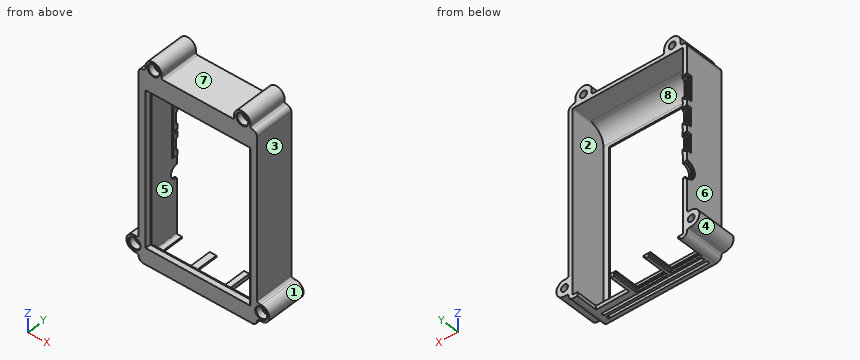
from build123d import *

# Parameters (mm, degrees)
BASE_DEPTH                      = 20.75
SHELL_T                         = -2
CLAMPS_DEPTH                    = 20.75
CLAMP_FILLETS_R                 = 1
SKETCH20_R                      = 1.8
CLAMP_HOLES_DEPTH               = 123.621878146
SKETCH21_R                      = 2.9
CLAMP_COUNTERSINKS_DEPTH        = 3.4
CLAMP_COUNTERSINK_CHAMFERS_SIZE = 0.3
SKETCH24_W                      = 14.5
SKETCH24_H                      = 12.8
USB_CUTOUT_DEPTH                = 18.25
SKETCH25_W                      = 16.5
SKETCH25_H                      = 13.5
USB_APPROACH_DEPTH              = 1.2
SKETCH28_W                      = 17.4
SKETCH28_H                      = 11.3
RJ45_CUTOUT_DEPTH               = 22.7
SKETCH29_W                      = 15
SKETCH29_H                      = 3.2
USB_C_SUPPORT_DEPTH             = 0.5
USB_C_SUPPORT_CHAMFER_SIZE      = 0.5
SKETCH30_W                      = 13
SKETCH30_H                      = 2.7
USB_C_APPROACH_DEPTH            = 1.5
USB_C_APPROACH_CHAMFER_SIZE     = 0.5
SKETCH36_W                      = 9.8
SKETCH36_H                      = 2.48
HDMI_APPROACH_DEPTH             = 1.5
HDMI_APPROACH_CHAMFER_SIZE      = 0.5
SKETCH37_W                      = 12.8
SKETCH37_H                      = 2.98
HDMI_SUPPORT_DEPTH              = 0.5
HDMI_SUPPORT_CHAMFER_SIZE       = 0.5
HDMI_CUTOUT_DEPTH               = 1
SKETCH32_R                      = 3.5
AUDIO_CUTOUT_DEPTH              = 2
SKETCH33_R                      = 4.75
AUDIO_APPROACH_DEPTH            = 1
AUDIO_APPROACH_CHAMFER_SIZE     = 0.5
AIR_SCOOP_REACH                 = 123.517
SKETCH41_W                      = 53
SKETCH41_H                      = 1.5
VENT_DEPTH                      = 2
VENT_FILLET_R                   = 0.5
SKETCH40_W                      = 52
SKETCH40_H                      = 78
SCREEN_CUTOUT_DEPTH             = 123.621878163
CHAMFER1_SIZE                   = 1.5


with BuildPart() as part:
    # Sketch2 → Base (new body)
    with BuildSketch(Plane(origin=(0, 0, 0), x_dir=(1, 0, 0), z_dir=(0, 1, 0))):
        with BuildLine():
            Line((2.5, 0), (59.5, 0))
            ThreePointArc((59.5, 0), (61.267766953, 0.732233047), (62, 2.5))
            Line((62, 2.5), (62, 97.1))
            ThreePointArc((62, 97.1), (61.267766953, 98.867766953), (59.5, 99.6))
            Line((59.5, 99.6), (2.5, 99.6))
            ThreePointArc((2.5, 99.6), (0.732233047, 98.867766953), (0, 97.1))
            Line((0, 97.1), (0, 2.5))
            ThreePointArc((0, 2.5), (0.732233047, 0.732233047), (2.5, 0))
        make_face()
    extrude(amount=BASE_DEPTH)

    # Shell
    shell_openings = [part.faces().sort_by_distance(p)[0] for p in [
        (31, 20.75, -49.8),
    ]]
    offset(amount=SHELL_T, openings=shell_openings, kind=Kind.INTERSECTION)

    # Sketch14 → Clamps (add)
    with BuildSketch(Plane.XZ):
        with BuildLine():
            Line((-2.2, -87.6), (0, -87.6))
            Line((0, -87.6), (0, -96.1))
            Line((0, -96.1), (-2.2, -96.1))
            ThreePointArc((-2.2, -96.1), (-6.45, -91.85), (-2.2, -87.6))
        make_face()
        with BuildLine():
            Line((3.5, 2.2), (3.5, 0))
            Line((3.5, 0), (12, 0))
            Line((12, 0), (12, 2.2))
            ThreePointArc((12, 2.2), (7.75, 6.45), (3.5, 2.2))
        make_face()
        with BuildLine():
            Line((64.2, -87.6), (62, -87.6))
            Line((62, -87.6), (62, -96.1))
            Line((62, -96.1), (64.2, -96.1))
            ThreePointArc((64.2, -96.1), (68.45, -91.85), (64.2, -87.6))
        make_face()
        with BuildLine():
            Line((50, 0), (50, 2.2))
            ThreePointArc((50, 2.2), (54.25, 6.45), (58.5, 2.2))
            Line((58.5, 2.2), (58.5, 0))
            Line((58.5, 0), (50, 0))
        make_face()
    extrude(amount=-CLAMPS_DEPTH)

    # Clamp Fillets
    clamp_fillets_edges = [part.edges().sort_by_distance(p)[0] for p in [
        (0, 10.375, -96.1),
        (0, 10.375, -87.6),
        (3.5, 10.375, 0),
        (12, 10.375, 0),
        (62, 10.375, -87.6),
        (62, 10.375, -96.1),
        (50, 10.375, 0),
        (58.5, 10.375, 0),
    ]]
    fillet(clamp_fillets_edges, radius=CLAMP_FILLETS_R - 0.0001)  # a hair under: the kernel refuses the full size

    # Sketch20 → Clamp Holes (cut, through all)
    with BuildSketch(Plane.XZ):
        with Locations(Location((7.75, 2.2, 0), (0, 0, 270))):
            Circle(SKETCH20_R)
        with Locations(Location((54.25, 2.2, 0), (0, 0, 270))):
            Circle(SKETCH20_R)
        with Locations(Location((64.2, -91.85, 0), (0, 0, 270))):
            Circle(SKETCH20_R)
        with Locations(Location((-2.2, -91.85, 0), (0, 0, 270))):
            Circle(SKETCH20_R)
    extrude(amount=-CLAMP_HOLES_DEPTH, mode=Mode.SUBTRACT)

    # Sketch21 → Clamp Countersinks (cut)
    with BuildSketch(Plane.XZ):
        with Locations(Location((7.75, 2.2, 0), (0, 0, 270))):
            Circle(SKETCH21_R)
        with Locations(Location((54.25, 2.2, 0), (0, 0, 270))):
            Circle(SKETCH21_R)
        with Locations(Location((64.2, -91.85, 0), (0, 0, 270))):
            Circle(SKETCH21_R)
        with Locations(Location((-2.2, -91.85, 0), (0, 0, 270))):
            Circle(SKETCH21_R)
    extrude(amount=-CLAMP_COUNTERSINKS_DEPTH, mode=Mode.SUBTRACT)

    # Clamp Countersink Chamfers
    clamp_countersink_chamfers_edges = [part.edges().sort_by_distance(p)[0] for p in [
        (-2.2, 0, -88.95),
        (64.2, 0, -88.95),
        (54.25, 0, 5.1),
        (7.75, 0, 5.1),
    ]]
    chamfer(clamp_countersink_chamfers_edges, length=CLAMP_COUNTERSINK_CHAMFERS_SIZE)

    # Sketch24 → USB Cutout (cut)
    with BuildSketch(Plane(origin=(0, 0, -99.6), x_dir=(-1, 0, 0), z_dir=(0, 0, -1))):
        with Locations((-30, 14.35)):
            Rectangle(SKETCH24_W, SKETCH24_H)
        with Locations((-12, 14.35)):
            Rectangle(SKETCH24_W, SKETCH24_H)
    extrude(amount=-USB_CUTOUT_DEPTH, mode=Mode.SUBTRACT)

    # Sketch25 → USB Approach (cut)
    with BuildSketch(Plane(origin=(0, 0, -99.6), x_dir=(-1, 0, 0), z_dir=(0, 0, -1))):
        with Locations((-30, 14)):
            Rectangle(SKETCH25_W, SKETCH25_H)
        with Locations((-12, 14)):
            Rectangle(SKETCH25_W, SKETCH25_H)
    extrude(amount=-USB_APPROACH_DEPTH, mode=Mode.SUBTRACT)

    # Sketch28 → RJ45 Cutout (cut)
    with BuildSketch(Plane(origin=(0, 0, -99.6), x_dir=(-1, 0, 0), z_dir=(0, 0, -1))):
        with Locations((-48.75, 15.1)):
            Rectangle(SKETCH28_W, SKETCH28_H)
    extrude(amount=-RJ45_CUTOUT_DEPTH, mode=Mode.SUBTRACT)

    # Sketch29 → USB-C Support (add)
    with BuildSketch(Plane(origin=(2, 0, 0), x_dir=(0, 0, -1), z_dir=(1, 0, 0))):
        with Locations((22.55, 19.15)):
            Rectangle(SKETCH29_W, SKETCH29_H)
    extrude(amount=USB_C_SUPPORT_DEPTH)

    # USB-C Support Chamfer
    usb_c_support_chamfer_edges = [part.edges().sort_by_distance(p)[0] for p in [
        (2.5, 19.15, -30.05),
        (2.5, 17.55, -22.55),
        (2.5, 19.15, -15.05),
    ]]
    chamfer(usb_c_support_chamfer_edges, length=USB_C_SUPPORT_CHAMFER_SIZE - 0.0001)  # a hair under: the kernel refuses the full size

    # Sketch30 → USB-C Approach (cut)
    with BuildSketch(Plane.ZY):
        with Locations((-22.55, 19.4)):
            Rectangle(SKETCH30_W, SKETCH30_H)
    extrude(amount=-USB_C_APPROACH_DEPTH, mode=Mode.SUBTRACT)

    # USB-C Approach Chamfer
    usb_c_approach_chamfer_edges = [part.edges().sort_by_distance(p)[0] for p in [
        (1.5, 19.4, -29.05),
        (1.5, 19.4, -16.05),
        (1.5, 18.05, -22.55),
    ]]
    chamfer(usb_c_approach_chamfer_edges, length=USB_C_APPROACH_CHAMFER_SIZE)

    # Sketch36 → HDMI Approach (cut)
    with BuildSketch(Plane.ZY):
        with Locations((-50.85, 19.51)):
            Rectangle(SKETCH36_W, SKETCH36_H)
        with Locations((-37.35, 19.51)):
            Rectangle(SKETCH36_W, SKETCH36_H)
    extrude(amount=-HDMI_APPROACH_DEPTH, mode=Mode.SUBTRACT)

    # HDMI Approach Chamfer
    hdmi_approach_chamfer_edges = [part.edges().sort_by_distance(p)[0] for p in [
        (1.5, 19.51, -55.75),
        (1.5, 19.51, -45.95),
        (1.5, 18.27, -50.85),
        (1.5, 19.51, -42.25),
        (1.5, 19.51, -32.45),
        (1.5, 18.27, -37.35),
    ]]
    chamfer(hdmi_approach_chamfer_edges, length=HDMI_APPROACH_CHAMFER_SIZE)

    # Sketch37 → HDMI Support (add)
    with BuildSketch(Plane(origin=(2, 0, 0), x_dir=(0, 0, -1), z_dir=(1, 0, 0))):
        with Locations((37.35, 19.26)):
            Rectangle(SKETCH37_W, SKETCH37_H)
        with Locations((50.85, 19.26)):
            Rectangle(SKETCH37_W, SKETCH37_H)
    extrude(amount=HDMI_SUPPORT_DEPTH)

    # HDMI Support Chamfer
    hdmi_support_chamfer_edges = [part.edges().sort_by_distance(p)[0] for p in [
        (2.5, 19.26, -57.25),
        (2.5, 17.77, -50.85),
        (2.5, 19.26, -44.45),
        (2.5, 19.26, -43.75),
        (2.5, 17.77, -37.35),
        (2.5, 19.26, -30.95),
    ]]
    chamfer(hdmi_support_chamfer_edges, length=HDMI_SUPPORT_CHAMFER_SIZE - 0.0001)  # a hair under: the kernel refuses the full size

    # Sketch38 → HDMI Cutout (cut)
    with BuildSketch(Plane.ZY.offset(-1.5)):
        with BuildLine():
            Line((-54.25, 20.75), (-47.45, 20.75))
            Line((-47.45, 20.75), (-47.45, 20.67))
            ThreePointArc((-47.45, 20.67), (-47.713603897, 20.033603897), (-48.35, 19.77))
            Line((-48.35, 19.77), (-53.35, 19.77))
            ThreePointArc((-53.35, 19.77), (-53.986396103, 20.033603897), (-54.25, 20.67))
            Line((-54.25, 20.67), (-54.25, 20.75))
        make_face()
        with BuildLine():
            Line((-40.75, 20.75), (-33.95, 20.75))
            Line((-33.95, 20.75), (-33.95, 20.67))
            ThreePointArc((-33.95, 20.67), (-34.213603897, 20.033603897), (-34.85, 19.77))
            Line((-34.85, 19.77), (-39.85, 19.77))
            ThreePointArc((-39.85, 19.77), (-40.486396103, 20.033603897), (-40.75, 20.67))
            Line((-40.75, 20.67), (-40.75, 20.75))
        make_face()
        with BuildLine():
            Line((-27.55, 20.75), (-17.55, 20.75))
            Line((-17.55, 20.75), (-17.55, 20.713167547))
            ThreePointArc((-17.55, 20.713167547), (-17.890683887, 19.890683887), (-18.713167547, 19.55))
            Line((-18.713167547, 19.55), (-26.386832453, 19.55))
            ThreePointArc((-26.386832453, 19.55), (-27.209316113, 19.890683887), (-27.55, 20.713167547))
            Line((-27.55, 20.713167547), (-27.55, 20.75))
        make_face()
    extrude(amount=-HDMI_CUTOUT_DEPTH, mode=Mode.SUBTRACT)

    # Sketch32 → Audio Cutout (cut)
    with BuildSketch(Plane.ZY):
        with Locations((-65.35, 20.75)):
            Circle(SKETCH32_R)
    extrude(amount=-AUDIO_CUTOUT_DEPTH, mode=Mode.SUBTRACT)

    # Sketch33 → Audio Approach (cut)
    with BuildSketch(Plane.ZY):
        with Locations((-65.35, 20.75)):
            Circle(SKETCH33_R)
    extrude(amount=-AUDIO_APPROACH_DEPTH, mode=Mode.SUBTRACT)

    # Audio Approach Chamfer
    audio_approach_chamfer_edges = [part.edges().sort_by_distance(p)[0] for p in [
        (1, 16, -65.35),
    ]]
    chamfer(audio_approach_chamfer_edges, length=AUDIO_APPROACH_CHAMFER_SIZE)

    # Air Scoop: up to this face of the body (flat: up to its plane)
    air_scoop_end = Plane(part.part.faces().sort_by_distance((2, 10.683962064, -50.685539842))[0])
    # Sketch39 → Air Scoop (add, up to the picked face)
    with BuildSketch(Plane.ZY.offset(-60), mode=Mode.PRIVATE) as air_scoop_sk1:
        with BuildLine():
            Line((-2, 2), (-10, 2))
            ThreePointArc((-10, 2), (-4.343145751, 4.343145751), (-2, 10))
            Line((-2, 10), (-2, 2))
        make_face()
    air_scoop_tool1 = split(extrude(air_scoop_sk1.sketch, amount=AIR_SCOOP_REACH, mode=Mode.PRIVATE), bisect_by=air_scoop_end, keep=Keep.BOTH, mode=Mode.PRIVATE)
    add(air_scoop_tool1.solids().sort_by(Axis((60, 3.786944, -3.786944), (-1, 0, 0)))[0])

    # Sketch41 → Vent (cut)
    with BuildSketch(Plane(origin=(0, 0, -99.6), x_dir=(-1, 0, 0), z_dir=(0, 0, -1))):
        with Locations((-31, 5.5)):
            Rectangle(SKETCH41_W, SKETCH41_H)
        with Locations((-31, 2.75)):
            Rectangle(SKETCH41_W, SKETCH41_H)
    extrude(amount=-VENT_DEPTH, mode=Mode.SUBTRACT)

    # Vent Fillet
    vent_fillet_edges = [part.edges().sort_by_distance(p)[0] for p in [
        (57.5, 4.75, -98.6),
        (57.5, 6.25, -98.6),
        (4.5, 6.25, -98.6),
        (4.5, 4.75, -98.6),
        (57.5, 2, -98.6),
        (57.5, 3.5, -98.6),
        (4.5, 3.5, -98.6),
        (4.5, 2, -98.6),
    ]]
    fillet(vent_fillet_edges, radius=VENT_FILLET_R)

    # Sketch40 → Screen Cutout (cut, through all)
    with BuildSketch(Plane.XZ):
        with Locations((31, -50.58226)):
            Rectangle(SKETCH40_W, SKETCH40_H)
    extrude(amount=-SCREEN_CUTOUT_DEPTH, mode=Mode.SUBTRACT)

    # Chamfer1
    chamfer1_edges = [part.edges().sort_by_distance(p)[0] for p in [
        (5, 0, -50.58226),
        (31, 0, -89.58226),
        (57, 0, -50.58226),
        (31, 0, -11.58226),
    ]]
    chamfer(chamfer1_edges, length=CHAMFER1_SIZE)


solid = part.part
Source: CAD feature listing. Evaluate the final solid. Frame: model axes, mm. Face numbers are marked on the shaded views. A direction names the side the tool comes from. Round coordinates to 2 decimals unless told otherwise and drop trailing zeros. Order: outer loops, then holes, each group sorted by start corner. A loop starts at its lowest first (then second) coordinate and runs counter-clockwise, first axis right, second up. Notation, with made-up numbers: (63, 66) - (110, 66) arc R18 cw to (110, 87) - close; hole circle Ø2 at (84.25, 29.25). An arc over 180 degrees is marked (long way). Use a Markdown table: item, result. Add a question column.
1. Section query D-D (x = 31.5). Return the cut outline in (y, z), then the cut area to 3 significant figures.
2. Section query A-A (x = 54.25). Give the number of separate pieces and of enclosed holes in the cut face, then the cut area to 3 significant figures.
3. Line query: probe 1 along X at (y, z) = (14.75, -91.85); probe 2 along X at (y, z) = (2.2, 2.2); probe 3 along X at (y, z) = (14.25, -47). Output: solid intervals per line, ascending.
4. Mould query, pull axis Z, two halves, no side actions, for the marked faces 1, 2 and 3. Classes: +Z half, -Z half, draft (parallel to the pull), parting line (faces both ways), or undercut.
5. First-contact query: pin 1 (1 mm diameter, centred on y = 13.5, z = -72.5, fed in from +X); pin 2 (1 mm diameter, centred on x = 60.5, y = 3.5, fed in from +Z); pin 3 (3.5 mm diameter, centred on x = 54.25, z = 2.2, fed in from -Y); pin 4 (0.8 mm diameter, centred on x = 0.5, z = -49, fed in from +Y). Flat tips, straight axial feed; report the tip coordinate or a pass-through.
6. Set-up query: the marked faces 4, 5, 6, 7 and 8. Return all of +Z, -Z, +X, -X, +Y, -Y with unobstructed straight access to the full face (end or side cutting, diameter ignored); none if empty.
Derived:
| question | item | result |
|---|---|---|
| 1 | outline | (0, -99.6) - (2, -99.6) - (2, -89.58) - (1.5, -89.58) - (0, -91.08) - close; (0, -10.08) - (1.5, -11.58) - (2, -11.58) - (2, -10) arc R8 cw to (10, -2) - (20.75, -2) - (20.75, 0) - (0, 0) - close; (3.5, -99.6) - (4.75, -99.6) - (4.75, -97.6) - (3.5, -97.6) - close; (6.25, -99.6) - (7.25, -99.6) - (7.25, -98.4) - (7.95, -98.4) - (7.95, -97.6) - (6.25, -97.6) - close |
| 1 | area | 97.2 mm2 |
| 2 | separate pieces | 5 |
| 2 | enclosed holes | 0 |
| 2 | area | 153 mm2 |
| 3 | probe 1 | -6.45 to -4, -0.4 to 2, 60 to 62.4, 66 to 68.45 |
| 3 | probe 2 | 3.5 to 4.85, 10.65 to 12, 50 to 51.35, 57.15 to 58.5 |
| 3 | probe 3 | 0 to 2, 60 to 62 |
| 4 | face 1 | parting line |
| 4 | face 2 | undercut |
| 4 | face 3 | draft |
| 5 | pin 1 | x = 62 |
| 5 | pin 2 | z = -0.05 |
| 5 | pin 3 | through |
| 5 | pin 4 | y = 18.27 |
| 6 | face 4 | -X, +Y, -Y |
| 6 | face 5 | none |
| 6 | face 6 | +Z, -X, +Y, -Y |
| 6 | face 7 | +Z, +Y, -Y |
| 6 | face 8 | +Y |
